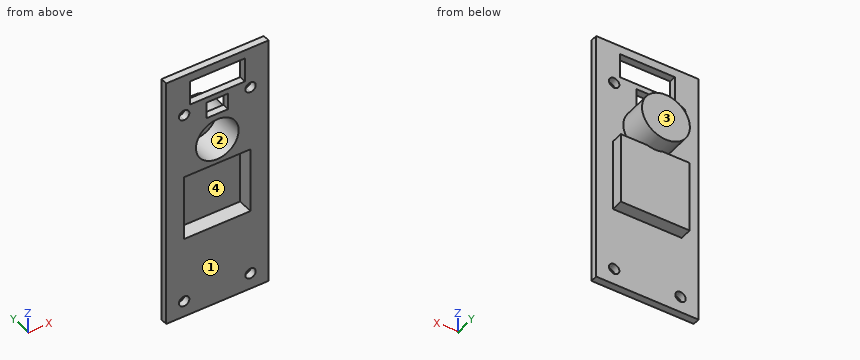
```python
from build123d import *

# Parameters (mm, degrees)
SKETCH1_W               = 29.4
SKETCH1_H               = 73.9
SKETCH1_W_2             = 15.82
SKETCH1_H_2             = 7.1
SKETCH1_W_3             = 6.2
SKETCH1_H_3             = 4.8
BOSS_EXTRUDE1_DEPTH     = 2
SKETCH1_3_R             = 6.875
BOSS_EXTRUDE2_DEPTH     = 10
SHELL1_T                = -0.75
SKETCH1_4_W             = 19.75
SKETCH1_4_H             = 20.75
BOSS_EXTRUDE3_DEPTH     = 5.4
SKETCH2_W               = 19
SKETCH2_H               = 19
CUT_EXTRUDE1_DEPTH      = 4.4
CUT_EXTRUDE2_DEPTH      = 41.563437971
CUT_EXTRUDE2_DEPTH_BACK = 41.563437971


with BuildPart() as part:
    # Sketch1 → Boss-Extrude1 (new body)
    with BuildSketch(Plane(origin=(0, 0, 0), x_dir=(1, 0, 0), z_dir=(0, 1, 0))):
        Rectangle(SKETCH1_W, SKETCH1_H)
        with Locations((0, -30.932)):
            Rectangle(SKETCH1_W_2, SKETCH1_H_2, mode=Mode.SUBTRACT)
        with Locations((0, -23.449)):
            Rectangle(SKETCH1_W_3, SKETCH1_H_3, mode=Mode.SUBTRACT)
        with BuildLine():
            Line((-9.875, 14.036), (9.875, 14.036))
            Line((9.875, 14.036), (9.875, -6.714))
            Line((9.875, -6.714), (2.239559108, -6.714))
            ThreePointArc((2.239559108, -6.714), (0, -20.089), (-2.239559108, -6.714))
            Line((-2.239559108, -6.714), (-9.875, -6.714))
            Line((-9.875, -6.714), (-9.875, 14.036))
        make_face(mode=Mode.SUBTRACT)
    extrude(amount=BOSS_EXTRUDE1_DEPTH)



with BuildPart() as body_2:
    # Sketch1<3> → Boss-Extrude2 (new body)
    with BuildSketch(Plane(origin=(0, 0, 0), x_dir=(1, 0, 0), z_dir=(0, 1, 0))):
        with Locations(Location((0, -13.214, 0), (0, 0, 270))):
            Circle(SKETCH1_3_R)
    extrude(amount=BOSS_EXTRUDE2_DEPTH)

    # Shell1
    shell1_openings = [body_2.faces().sort_by_distance(p)[0] for p in [
        (0, 0, 13.214),
    ]]
    offset(amount=SHELL1_T, openings=shell1_openings, kind=Kind.INTERSECTION)


with BuildPart() as part_1:
    add(part.part)

    add(body_2.part)  # Boss-Extrude3 merges body 2
    # Sketch1<4> → Boss-Extrude3 (add)
    with BuildSketch(Plane(origin=(0, 0, 0), x_dir=(1, 0, 0), z_dir=(0, 1, 0))):
        with Locations((0, 3.661)):
            Rectangle(SKETCH1_4_W, SKETCH1_4_H)
    extrude(amount=BOSS_EXTRUDE3_DEPTH)

    # Sketch2 → Cut-Extrude1 (cut)
    with BuildSketch(Plane.XZ):
        with Locations((0, -3.661)):
            Rectangle(SKETCH2_W, SKETCH2_H)
    extrude(amount=-CUT_EXTRUDE1_DEPTH, mode=Mode.SUBTRACT)

    # Sketch3 → Cut-Extrude2 (cut, two sides: drawn at the far end of the back side and taken through both)
    with BuildSketch(Plane(origin=(0, 2, 0), x_dir=(1, 0, 0), z_dir=(0, 1, 0)).offset(-CUT_EXTRUDE2_DEPTH_BACK)):
        with BuildLine():
            Line((-9.525, 30.775), (-9.525, 32.275))
            Line((-9.525, 32.275), (-8.025, 32.275))
            ThreePointArc((-8.025, 32.275), (-10.585660172, 33.335660172), (-9.525, 30.775))
        make_face()
        with BuildLine():
            Line((-8.025, 32.275), (-9.525, 32.275))
            Line((-9.525, 32.275), (-9.525, 30.775))
            ThreePointArc((-9.525, 30.775), (-8.464339828, 31.214339828), (-8.025, 32.275))
        make_face()
        with BuildLine():
            ThreePointArc((11.025, 32.275), (9.525, 33.775), (8.025, 32.275))
            Line((8.025, 32.275), (9.525, 32.275))
            Line((9.525, 32.275), (9.525, 30.775))
            ThreePointArc((9.525, 30.775), (10.585660172, 31.214339828), (11.025, 32.275))
        make_face()
        with BuildLine():
            Line((9.525, 32.275), (8.025, 32.275))
            ThreePointArc((8.025, 32.275), (8.464339828, 31.214339828), (9.525, 30.775))
            Line((9.525, 30.775), (9.525, 32.275))
        make_face()
        with BuildLine():
            ThreePointArc((11.025, -24.875), (10.585660172, -23.814339828), (9.525, -23.375))
            Line((9.525, -23.375), (9.525, -24.875))
            Line((9.525, -24.875), (8.025, -24.875))
            ThreePointArc((8.025, -24.875), (9.525, -26.375), (11.025, -24.875))
        make_face()
        with BuildLine():
            Line((9.525, -24.875), (9.525, -23.375))
            ThreePointArc((9.525, -23.375), (8.464339828, -23.814339828), (8.025, -24.875))
            Line((8.025, -24.875), (9.525, -24.875))
        make_face()
        with BuildLine():
            ThreePointArc((-8.025, -24.875), (-8.464339828, -23.814339828), (-9.525, -23.375))
            Line((-9.525, -23.375), (-9.525, -24.875))
            Line((-9.525, -24.875), (-8.025, -24.875))
        make_face()
        with BuildLine():
            Line((-9.525, -24.875), (-9.525, -23.375))
            ThreePointArc((-9.525, -23.375), (-10.585660172, -25.935660172), (-8.025, -24.875))
            Line((-8.025, -24.875), (-9.525, -24.875))
        make_face()
    extrude(amount=CUT_EXTRUDE2_DEPTH + CUT_EXTRUDE2_DEPTH_BACK, mode=Mode.SUBTRACT)


solid = part_1.part
```
Verification items for the finished model (mm, model axes). Face numbers are marked on the shaded views. A direction names the side the tool comes from. Round coordinates to 2 decimals unless told otherwise and drop trailing zeros. Write each loop counter-clockwise with the first axis right and the second up, starting at its lowest first coordinate (ties: lowest second). Pieces come first, ordered by that corner, then holes. Notation, with made-up numbers: (-16, 30.25) -> (19, 30.25) arc R16 ccw to (19, 53.25) -> close; hole circle Ø1 at (59, -21.75). An arc over 180 degrees is marked (long way). Write each question's results on one line, items separated by ' | '. Start each with the question number.
1. Depth check by flat-ended pin: P1, Ø3, axis at x = -9, z = 8, coming from the +Y side; P2, Ø1, axis at x = 8, y = 3.5, coming from the +Z side; P3, Ø1.7, axis at x = 2, y = 3.5, coming from the -Z side. Enter the tip coordinate at first touch or a pass-through.
2. Cross-section at D-D (x = 4.5). Enter the section's corners in (y, z), then the cut area to 3 significant figures.
3. Cross-section at A-A (x = 0). Enter the section's corners in (y, z), then the cut area to 3 significant figures.
4. Cross-section at C-C (z = -12). Enter the section's corners in (x, y) (3 decimals), then the cut area to 4 significant figures.
5. Draft check along X on the marked faces 1 and 2. Enter one of: +X half, -X half, draft (parallel to the pull), parting line (faces both ways), or undercut.
6. Material ranges on probe 1 along Z at (x, y) = (7, 0.5); probe 2 along X at (y, z) = (1.75, 2); probe 3 along Z at (x, y) = (-2, 3), recorded low to high. Write a range as from..to.
7. Cross-section at B-B (y = 3.5). Enter the section's corners in (x, z) (3 decimals).
8. Set-up check for the marked faces 3 and 4: record each of +Z, -Z, +X, -X, +Y, -Y from which the full face is reachable in a straight line by a thin tool's end or side.
Solutions:
1) P1: stops at y = 5.4 | P2: stops at z = 6.71 | P3: stops at z = -14.04
2) outline: (0, -36.95) -> (2, -36.95) -> (2, -14.04) -> (5.4, -14.04) -> (5.4, 6.71) -> (2, 6.71) -> (2, 8.02) -> (10, 8.02) -> (10, 18.41) -> (2, 18.41) -> (2, 27.38) -> (0, 27.38) -> (0, 17.37) -> (9.25, 17.37) -> (9.25, 9.06) -> (0, 9.06) -> (0, 5.84) -> (4.4, 5.84) -> (4.4, -13.16) -> (0, -13.16) -> close; (0, 34.48) -> (2, 34.48) -> (2, 36.95) -> (0, 36.95) -> close | area: 127 mm2
3) outline: (0, -36.95) -> (2, -36.95) -> (2, -14.04) -> (5.4, -14.04) -> (5.4, 6.34) -> (10, 6.34) -> (10, 20.09) -> (2, 20.09) -> (2, 21.05) -> (0, 21.05) -> (0, 19.34) -> (9.25, 19.34) -> (9.25, 7.09) -> (0, 7.09) -> (0, 5.84) -> (4.4, 5.84) -> (4.4, -13.16) -> (0, -13.16) -> close; (0, 25.85) -> (2, 25.85) -> (2, 27.38) -> (0, 27.38) -> close; (0, 34.48) -> (2, 34.48) -> (2, 36.95) -> (0, 36.95) -> close | area: 106 mm2
4) outline: (-14.7, 0) -> (-9.5, 0) -> (-9.5, 4.4) -> (9.5, 4.4) -> (9.5, 0) -> (14.7, 0) -> (14.7, 2) -> (9.875, 2) -> (9.875, 5.4) -> (-9.875, 5.4) -> (-9.875, 2) -> (-14.7, 2) -> close | area: 42.35 mm2
5) face 1: draft | face 2: undercut
6) probe 1: z = -36.95..-13.16, 5.84..27.38, 34.48..36.95 | probe 2: x = -14.7..-9.5, 9.5..14.7 | probe 3: z = -14.04..-13.16, 5.84..7.42, 19..19.79
7) outline: (-9.875, -14.036) -> (9.875, -14.036) -> (9.875, 6.714) -> (2.24, 6.714) arc R6.875 ccw (long way) to (-2.24, 6.714) -> (-9.875, 6.714) -> close; hole (-9.5, -13.161) -> (9.5, -13.161) -> (9.5, 5.839) -> (-9.5, 5.839) -> close; hole circle Ø12.25 at (0, 13.214)
8) face 3: +Z, -Z, +X, -X, +Y | face 4: -Y
